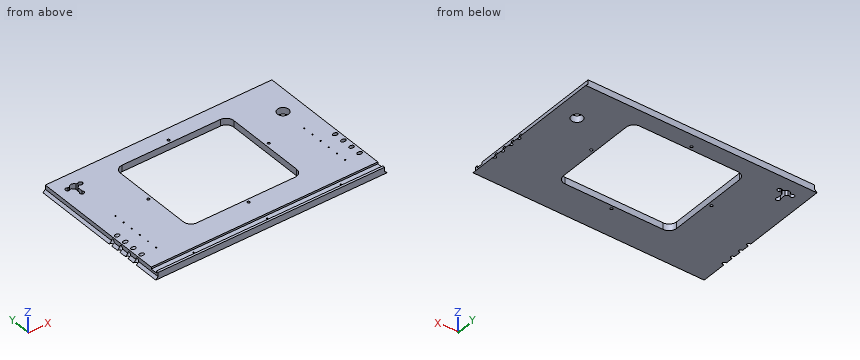
from build123d import *

# Parameters (mm, degrees)
CABFRONTOUTLINE_W               = 628.65
CABFRONTOUTLINE_H               = 396.08125
CABFRONT_THICKNESS_DEPTH        = 17.78
CABFRONT_COINDOORCUTS_R         = 1.5875
CUT_EXTRUDE1_DEPTH              = 12.7
SKETCH5_R                       = 15.08125
SKETCH5_R_2                     = 3.4925
SKETCH5_W                       = 308.0004
SKETCH5_H                       = 261.9629
CUT_EXTRUDE8_DEPTH              = 17.78
CABFRONTBOTTOMLEDGE_DEPTH_DEPTH = 5.08
CUT_EXTRUDE4_DEPTH              = 396.08125
FILLET1_R                       = 20.6502
SKETCH2_R                       = 4.7625
CUT_EXTRUDE5_DEPTH              = 76.2
SKETCH3_R                       = 4.7625
CUT_EXTRUDE6_DEPTH              = 76.2
SKETCH4_R                       = 4.7625
CUT_EXTRUDE7_DEPTH              = 76.2
SKETCH6_R                       = 4.7625
CUT_EXTRUDE9_DEPTH              = 76.2


with BuildPart() as part:
    # CabFrontOutline → CabFront_Thickness (new body)
    with BuildSketch(Plane.XY):
        with Locations((12009.966666666, -5854.303125)):
            Rectangle(CABFRONTOUTLINE_W, CABFRONTOUTLINE_H)
    extrude(amount=-CABFRONT_THICKNESS_DEPTH)

    # CabFront_CoinDoorCuts → Cut-Extrude1 (cut)
    with BuildSketch(Plane.XY):
        with Locations((11753.109166666, -5893.59375)):
            Circle(CABFRONT_COINDOORCUTS_R)
        with Locations((11753.109166666, -5950.74375)):
            Circle(CABFRONT_COINDOORCUTS_R)
        with Locations((12266.824166666, -5893.59375)):
            Circle(CABFRONT_COINDOORCUTS_R)
        with Locations((12266.824166666, -5950.74375)):
            Circle(CABFRONT_COINDOORCUTS_R)
        with Locations((11753.109166666, -5836.44375)):
            Circle(CABFRONT_COINDOORCUTS_R)
        with Locations((12266.824166666, -5836.44375)):
            Circle(CABFRONT_COINDOORCUTS_R)
        with Locations((12266.824166666, -5865.01875)):
            Circle(CABFRONT_COINDOORCUTS_R)
        with Locations((12266.824166666, -5922.16875)):
            Circle(CABFRONT_COINDOORCUTS_R)
        with Locations((12266.824166666, -5979.31875)):
            Circle(CABFRONT_COINDOORCUTS_R)
        with Locations((12209.991666666, -6037.10375)):
            Circle(CABFRONT_COINDOORCUTS_R)
        with Locations((12009.966666666, -6037.10375)):
            Circle(CABFRONT_COINDOORCUTS_R)
        with Locations((11809.941666666, -6037.10375)):
            Circle(CABFRONT_COINDOORCUTS_R)
        with Locations((11753.109166666, -5979.31875)):
            Circle(CABFRONT_COINDOORCUTS_R)
        with Locations((11753.109166666, -5922.16875)):
            Circle(CABFRONT_COINDOORCUTS_R)
        with Locations((11753.109166666, -5865.01875)):
            Circle(CABFRONT_COINDOORCUTS_R)
    extrude(amount=-CUT_EXTRUDE1_DEPTH, mode=Mode.SUBTRACT)

    # Sketch5 → Cut-Extrude8 (cut)
    with BuildSketch(Plane.XY):
        with Locations((12267.141666666, -5761.0375)):
            Circle(SKETCH5_R)
        with Locations((12173.479166666, -5831.68125)):
            Circle(SKETCH5_R_2)
        with Locations((11846.454166666, -5831.68125)):
            Circle(SKETCH5_R_2)
        with Locations((12009.966666666, -5972.175)):
            Circle(SKETCH5_R_2)
        with Locations((12009.966666666, -5691.1875)):
            Circle(SKETCH5_R_2)
        with Locations((12009.966666666, -5831.68125)):
            Rectangle(SKETCH5_W, SKETCH5_H)
        with BuildLine():
            Line((11734.654409808, -5693.754968556), (11739.23011943, -5693.754968556))
            ThreePointArc((11739.23011943, -5693.754968556), (11748.029166666, -5687.976468556), (11756.828213901, -5693.754968556))
            Line((11756.828213901, -5693.754968556), (11761.386355753, -5693.754968556))
            ThreePointArc((11761.386355753, -5693.754968556), (11767.531113043, -5692.357368906), (11771.079666666, -5697.564968556))
            ThreePointArc((11771.079666666, -5697.564968556), (11767.531113043, -5702.772568206), (11761.386355753, -5701.374968556))
            Line((11761.386355753, -5701.374968556), (11756.828213901, -5701.374968556))
            ThreePointArc((11756.828213901, -5701.374968556), (11754.760305425, -5704.393665595), (11751.712166666, -5706.417925308))
            Line((11751.712166666, -5706.417925308), (11751.712166666, -5721.30243896))
            ThreePointArc((11751.712166666, -5721.30243896), (11748.029166666, -5731.092968556), (11744.346166666, -5721.30243896))
            Line((11744.346166666, -5721.30243896), (11744.346166666, -5706.417925308))
            ThreePointArc((11744.346166666, -5706.417925308), (11741.298027907, -5704.393665595), (11739.23011943, -5701.374968556))
            Line((11739.23011943, -5701.374968556), (11734.654409809, -5701.374968556))
            ThreePointArc((11734.654409809, -5701.374968556), (11724.978666666, -5697.564968556), (11734.654409808, -5693.754968556))
        make_face()
    extrude(amount=-CUT_EXTRUDE8_DEPTH, mode=Mode.SUBTRACT)

    # CabFront_BottomLedge → CabFrontBottomLedge_Depth (cut)
    with BuildSketch(Plane.XY):
        Polygon((11975.041666666, -6028.21375), (11695.641666666, -6028.21375), (11695.641666666, -6045.99375), (12324.291666666, -6045.99375), (12324.291666666, -6028.21375), align=None)
    extrude(amount=-CABFRONTBOTTOMLEDGE_DEPTH_DEPTH, mode=Mode.SUBTRACT)

    # CabFront_EdgeBevel → Cut-Extrude4 (cut)
    with BuildSketch(Plane.XZ.offset(6052.34375)):
        Polygon((11701.991666666, -11.43), (11701.991666666, 0), (11695.641666666, 0), (11695.641666666, -17.78), align=None)
        Polygon((12317.941666666, -11.43), (12324.291666666, -17.78), (12324.291666666, 0), (12317.941666666, 0), align=None)
    extrude(amount=-CUT_EXTRUDE4_DEPTH, mode=Mode.SUBTRACT)

    # Fillet1
    fillet1_edges = [part.edges().sort_by_distance(p)[0] for p in [
        (11855.966466666, -5962.6627, -8.89),
        (11855.966466666, -5700.6998, -8.89),
        (12163.966866666, -5700.6998, -8.89),
        (12163.966866666, -5962.6627, -8.89),
    ]]
    fillet(fillet1_edges, radius=FILLET1_R)

    # Sketch2 → Cut-Extrude5 (cut)
    with BuildSketch(Plane(origin=(5872.794384557, 0, 5872.794384557), x_dir=(0.707106781, 0, -0.707106781), z_dir=(0.707106781, 0, 0.707106781))):
        with Locations((8282.639891397, -5922.16875)):
            Circle(SKETCH2_R)
        with Locations((8282.639891397, -5979.31875)):
            Circle(SKETCH2_R)
    extrude(amount=-CUT_EXTRUDE5_DEPTH, mode=Mode.SUBTRACT)

    # Sketch3 → Cut-Extrude6 (cut)
    with BuildSketch(Plane(origin=(6137.172282109, 0, -6137.172282109), x_dir=(0.707106781, 0, 0.707106781), z_dir=(-0.707106781, 0, 0.707106781))):
        with Locations((8702.017852251, -5922.16875)):
            Circle(SKETCH3_R)
        with Locations((8702.017852251, -5979.31875)):
            Circle(SKETCH3_R)
    extrude(amount=-CUT_EXTRUDE6_DEPTH, mode=Mode.SUBTRACT)

    # Sketch4 → Cut-Extrude7 (cut)
    with BuildSketch(Plane(origin=(6137.165932109, 0, -6137.165932109), x_dir=(0.707106781, 0, 0.707106781), z_dir=(-0.707106781, 0, 0.707106781))):
        with Locations((8702.008871995, -5950.74375)):
            Circle(SKETCH4_R)
        with Locations((8702.008871995, -5893.59375)):
            Circle(SKETCH4_R)
    extrude(amount=-CUT_EXTRUDE7_DEPTH, mode=Mode.SUBTRACT)

    # Sketch6 → Cut-Extrude9 (cut)
    with BuildSketch(Plane(origin=(5872.800734557, 0, 5872.800734557), x_dir=(0.707106781, 0, -0.707106781), z_dir=(0.707106781, 0, 0.707106781))):
        with Locations((8282.648871653, -5893.59375)):
            Circle(SKETCH6_R)
        with Locations((8282.648871653, -5950.74375)):
            Circle(SKETCH6_R)
    extrude(amount=-CUT_EXTRUDE9_DEPTH, mode=Mode.SUBTRACT)


solid = part.part
Source: CAD feature listing. Evaluate the final solid. Frame: model axes, mm. Coordinates: 2 decimals unless noted, no trailing zeros. Loops run counter-clockwise (first coordinate to the right, second up) from the corner with the lowest first, then second, coordinate; pieces in that order, holes last. Notation, with made-up numbers: (-35.75, 35) -> (-25.75, 35) arc R29 ccw to (-25.75, 62) -> close; hole circle Ø2 at (-36.75, 3.25). An arc over 180 degrees is marked (long way). Answer in a Markdown table with one row per item. Add a question column.
Q1. Contact query for flat-ended pins moving along their axis: pin 1 Ø6.5 at (x, y) = (12009.97, -5691.19) entering from +Z; pin 2 Ø9 at (y, z) = (-5871.5, -3.5) entering from +X; pin 3 Ø1.6 at (x, y) = (11752.5, -5836.5) entering from +Z; pin 4 Ø2.5 at (x, y) = (12210, -6036.5) entering from +Z. Output: stop coordinate, or through.
Q2. Section B-B on x = 12102.5. Return the cut outline in (y, z).
Q3. Section A-A on y = -5819.5. Return the cut outline in (x, z), and give its area (3 significant figures).
Q4. Section D-D on x = 12259. Return the cut outline in (y, z), and give its area (3 significant figures).
Q5. Section C-C on y = -6017. Return the cut outline in (x, z).
Q6. Ray query, line 1 along X through (y, z) = (-5748, -10.75); line 2 along Y through (x, z) = (12087, -3.5); line 3 along Y through (x, z) = (12048, -8.75). Return the intervals inside material, ascending.
Computed values:
| question | item | result |
|---|---|---|
| 1 | pin 1 | passes through |
| 1 | pin 2 | stops at x = 12317.94 |
| 1 | pin 3 | stops at z = -12.7 |
| 1 | pin 4 | stops at z = -5.08 |
| 2 | outline | (-6052.34, -17.78) -> (-5962.66, -17.78) -> (-5962.66, 0) -> (-6028.21, 0) -> (-6028.21, -5.08) -> (-6045.99, -5.08) -> (-6045.99, 0) -> (-6052.34, 0) -> close; (-5700.7, -17.78) -> (-5656.26, -17.78) -> (-5656.26, 0) -> (-5700.7, 0) -> close |
| 3 | outline | (11695.64, -17.78) -> (11855.97, -17.78) -> (11855.97, 0) -> (11701.99, 0) -> (11701.99, -11.43) -> close; (12163.97, -17.78) -> (12324.29, -17.78) -> (12317.94, -11.43) -> (12317.94, 0) -> (12163.97, 0) -> close |
| 3 | area | 5,520 mm^2 |
| 4 | outline | (-6052.34, -17.78) -> (-5773.73, -17.78) -> (-5773.73, 0) -> (-6028.21, 0) -> (-6028.21, -5.08) -> (-6045.99, -5.08) -> (-6045.99, 0) -> (-6052.34, 0) -> close; (-5748.34, -17.78) -> (-5656.26, -17.78) -> (-5656.26, 0) -> (-5748.34, 0) -> close |
| 4 | area | 6,500 mm^2 |
| 5 | outline | (11695.64, -17.78) -> (12324.29, -17.78) -> (12317.94, -11.43) -> (12317.94, 0) -> (11701.99, 0) -> (11701.99, -11.43) -> close |
| 6 | line 1 | x = 11701.99 to 11855.97, 12163.97 to 12259.56, 12274.72 to 12317.94 |
| 6 | line 2 | y = -6052.34 to -6045.99, -6028.21 to -5962.66, -5700.7 to -5656.26 |
| 6 | line 3 | y = -6052.34 to -5962.66, -5700.7 to -5656.26 |
